Read the model definition and answer for the solid it produces. Units are mm, in the model's axes. Face numbers are marked on the shaded views. A direction names the side the tool comes from. Coordinates: 2 decimals unless noted, no trailing zeros. Loops run counter-clockwise (first coordinate to the right, second up) from the corner with the lowest first, then second, coordinate; pieces in that order, holes last. Notation, with made-up numbers: M 8,59 L 43,59 A19 ccw 43,71 Z; hole C 57,69 d7. An arc over 180 degrees is marked long. Put each result on its own line as item: value.
from build123d import *

# Parameters (mm, degrees)
EXTRUDE_1_DEPTH     = 55
EXTRUDE_2_DEPTH     = 55
EXTRUDE_3_DEPTH     = 2.7
EXTRUDE_START       = 52.3
EXTRUDE_4_DEPTH     = 2.7
SKETCH_4_W          = 25.5
SKETCH_4_H          = 18
SKETCH_4_W_2        = 29
SKETCH_4_H_2        = 10
CUT_EXTRUDE_1_DEPTH = 2.7


with BuildPart() as part:
    # Sketch 2 → Extrude 1 (new body)
    with BuildSketch(Plane.XY.offset(-27.5)):
        Polygon((57.3, 217.3), (57.3, 157), (60, 157), (60, 220), (-60, 220), (-60, 157), (-57.3, 157), (-57.3, 217.3), align=None)
    extrude(amount=EXTRUDE_1_DEPTH)



with BuildPart() as body_2:
    # Sketch 2_7 → Extrude 2 (new body)
    with BuildSketch(Plane.XY.offset(-27.5)):
        Polygon((57.3, 63), (60, 63), (60, 0), (-60, 0), (-60, 63), (-57.3, 63), (-57.3, 2.7), (57.3, 2.7), align=None)
    extrude(amount=EXTRUDE_2_DEPTH)


with BuildPart() as part_1:
    add(part.part)

    add(body_2.part)  # Extrude 3 merges body 2
    # Sketch 2_8 → Extrude 3 (add)
    with BuildSketch(Plane.XY.offset(-27.5)):
        Polygon((57.3, 157), (60, 157), (13.185508624, 110), (60, 63), (57.3, 63), (57.3, 2.7), (-57.3, 2.7), (-57.3, 63), (-60, 63), (-13.185508624, 110), (-60, 157), (-57.3, 157), (-57.3, 217.3), (57.3, 217.3), align=None)
        Polygon((46, 157), (-0.18191994, 111.000359728), (-46, 157), (0.18191994, 202.999640272), align=None, mode=Mode.SUBTRACT)
        Polygon((46, 63), (-0.18191994, 108.999640272), (-46, 63), (0.18191994, 17.000359728), align=None, mode=Mode.SUBTRACT)
    extrude(amount=EXTRUDE_3_DEPTH)

    # Sketch 2_9 → Extrude 4 (add)
    with BuildSketch(Plane.XY.offset(-27.5).offset(EXTRUDE_START)):
        Polygon((57.3, 157), (60, 157), (13.185508624, 110), (60, 63), (57.3, 63), (57.3, 2.7), (-57.3, 2.7), (-57.3, 63), (-60, 63), (-13.185508624, 110), (-60, 157), (-57.3, 157), (-57.3, 217.3), (57.3, 217.3), align=None)
        Polygon((46, 157), (-0.18191994, 111.000359728), (-46, 157), (0.18191994, 202.999640272), align=None, mode=Mode.SUBTRACT)
        Polygon((46, 63), (-0.18191994, 108.999640272), (-46, 63), (0.18191994, 17.000359728), align=None, mode=Mode.SUBTRACT)
    extrude(amount=EXTRUDE_4_DEPTH)

    # Sketch 4 → Cut-Extrude 1 (cut)
    with BuildSketch(Plane(origin=(60, 0, 0), x_dir=(0, 0, -1), z_dir=(1, 0, 0))):
        with Locations((0.25, 39)):
            Rectangle(SKETCH_4_W, SKETCH_4_H)
        with Locations((0, 58)):
            Rectangle(SKETCH_4_W_2, SKETCH_4_H_2)
    extrude(amount=-CUT_EXTRUDE_1_DEPTH, mode=Mode.SUBTRACT)


solid = part_1.part
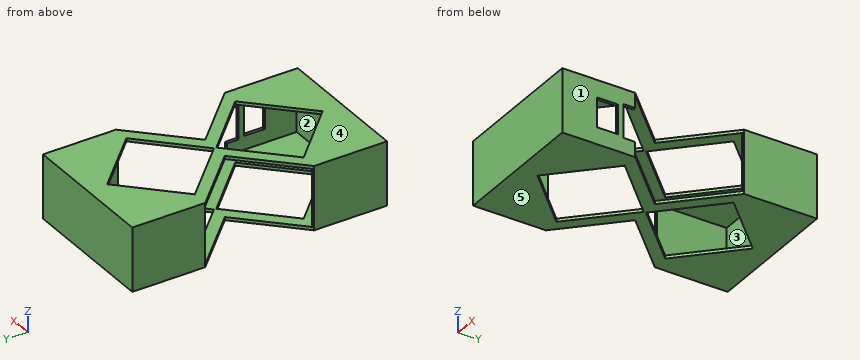
1) Given pin 1 Ø10 at (x, z) = (31.5, 14.5) entering from -Y, flat-ended and moving along its own axis, determine where the tip first touches the part or whether it passes through.
Answer list:
pin 1: stops at y = 0
2) Find section D-D, the plane y = 120. Write down the section's boundary in (x, z).
Answer list:
outline: M -23.15,-27.5 L -9.15,-27.5 L -9.15,-24.8 L -23.15,-24.8 Z; M -23.15,24.8 L -9.15,24.8 L -9.15,27.5 L -23.15,27.5 Z; M 8.85,-27.5 L 23.15,-27.5 L 23.15,-24.8 L 8.85,-24.8 Z; M 8.85,24.8 L 23.15,24.8 L 23.15,27.5 L 8.85,27.5 Z
3) Find section A-A, the plane z = -3.5. Write down the section's boundary in (x, y), plus the area to 3 significant figures.
Answer list:
outline: M -60,0 L 60,0 L 60,30 L 57.3,30 L 57.3,2.7 L -57.3,2.7 L -57.3,63 L -60,63 Z; M -60,157 L -57.3,157 L -57.3,217.3 L 57.3,217.3 L 57.3,157 L 60,157 L 60,220 L -60,220 Z; M 57.3,48 L 60,48 L 60,53 L 57.3,53 Z
area: 1,220 mm^2
4) Straight lines are drawn through the part: line 1 (Y direction, x = 41, z = -23.5); line 2 (X direction, y = 18.5, z = -2); line 3 (Z direction, x = -36.5, y = 29). For each, find the intervals that lie inside material, in ascending order. Write a range as [from, to].
Answer list:
line 1: y = [0, 2.7], [217.3, 220]
line 2: x = [-60, -57.3], [57.3, 60]
line 3: z = [-27.5, -24.8], [24.8, 27.5]
5) Find section B-B, the plane z = 22.5. Write down the section's boundary in (x, y).
Answer list:
outline: M -60,0 L 60,0 L 60,63 L 57.3,63 L 57.3,2.7 L -57.3,2.7 L -57.3,63 L -60,63 Z; M -60,157 L -57.3,157 L -57.3,217.3 L 57.3,217.3 L 57.3,157 L 60,157 L 60,220 L -60,220 Z
6) Determine the mould class of the marked faces 3, 4 and 5 for opening direction Z: released by +Z, released by -Z, zero draft, split by the parting line, or undercut.
Answer list:
face 3: undercut
face 4: released by +Z
face 5: released by -Z
7) Find section C-C, the plane y = 168.5. Write down the section's boundary in (x, z), plus the area to 3 significant figures.
Answer list:
outline: M -60,-27.5 L -34.45,-27.5 L -34.45,-24.8 L -57.3,-24.8 L -57.3,24.8 L -34.45,24.8 L -34.45,27.5 L -60,27.5 Z; M 34.55,-27.5 L 60,-27.5 L 60,27.5 L 34.55,27.5 L 34.55,24.8 L 57.3,24.8 L 57.3,-24.8 L 34.55,-24.8 Z
area: 543 mm^2
8) Which of the six approach directions +Z, -Z, +X, -X, +Y, -Y give full straight-line access (tool end or side, diameter ignored) to the marked faces 1 and 2?
Answer list:
face 1: +Z, -Z, +X, +Y, -Y
face 2: none
